Source: CAD feature listing. Evaluate the final solid. Frame: model axes, mm. Face numbers are marked on the shaded views. A direction names the side the tool comes from. Round coordinates to 2 decimals unless told otherwise and drop trailing zeros. Loops run counter-clockwise (first coordinate to the right, second up) from the corner with the lowest first, then second, coordinate; pieces in that order, holes last. Notation, with made-up numbers: M 89,-10.5 L 115,-10.5 A16 cw 115,8.5 Z; hole C 32.5,81 d6. An arc over 180 degrees is marked long. Answer as a JSON object with one key per item and string values.
from build123d import *

# Parameters (mm, degrees)
SKETCH1_W                       = 36
SKETCH1_H                       = 36
BOSS_EXTRUDE1_DEPTH             = 13.5
SKETCH1_3_W                     = 40
SKETCH1_3_H                     = 48.5
SKETCH1_3_W_2                   = 36
SKETCH1_3_H_2                   = 36
BOSS_EXTRUDE2_DEPTH             = 10
FILLET1_R                       = 3.5
FILLET2_R                       = 3.5
FILLET3_R                       = 1
FILLET4_R                       = 1
FILLET5_R                       = 1
BOSS_EXTRUDE3_REACH             = 39.343
BOSS_EXTRUDE3_DIRECTION_2_REACH = 39.343
BOSS_EXTRUDE4_REACH             = 41.68
BOSS_EXTRUDE4_DIRECTION_2_REACH = 41.68
BOSS_EXTRUDE5_DEPTH             = 12.5
SKETCH9_R                       = 2
CUT_EXTRUDE3_DEPTH              = 71.944630699
FILLET6_R                       = 1
FILLET7_R                       = 1


with BuildPart() as part:
    # Sketch1 → Boss-Extrude1 (new body)
    with BuildSketch(Plane.XY):
        Rectangle(SKETCH1_W, SKETCH1_H)
    extrude(amount=BOSS_EXTRUDE1_DEPTH)

    # Fillet2
    fillet2_edges = [part.edges().sort_by_distance(p)[0] for p in [
        (-18, 18, 6.75),
        (-18, -18, 6.75),
        (18, -18, 6.75),
        (18, 18, 6.75),
    ]]
    fillet(fillet2_edges, radius=FILLET2_R)

    # Fillet5
    fillet5_edges = [part.edges().sort_by_distance(p)[0] for p in [
        (0, 18, 13.5),
        (18, 0, 13.5),
        (-18, 0, 13.5),
        (0, -18, 13.5),
        (-16.974873734, 16.974873734, 13.5),
        (-16.974873734, -16.974873734, 13.5),
        (16.974873734, -16.974873734, 13.5),
        (16.974873734, 16.974873734, 13.5),
    ]]
    fillet(fillet5_edges, radius=FILLET5_R)


with BuildPart() as body_2:
    # Sketch1_3 → Boss-Extrude2 (new body)
    # profile 1 of 2: a face of its own
    with BuildSketch(Plane.XY):
        with Locations((0, -4.25)):
            Rectangle(SKETCH1_3_W, SKETCH1_3_H)
        Rectangle(SKETCH1_3_W_2, SKETCH1_3_H_2, mode=Mode.SUBTRACT)
    # profile 2 of 2: a face of its own
    with BuildSketch(Plane.XY):
        Rectangle(SKETCH1_3_W_2, SKETCH1_3_H_2)
    extrude(amount=-BOSS_EXTRUDE2_DEPTH)

    # Fillet1
    fillet1_edges = [body_2.edges().sort_by_distance(p)[0] for p in [
        (20, -28.5, -5),
        (-20, -28.5, -5),
        (-20, 20, -5),
        (20, 20, -5),
    ]]
    fillet(fillet1_edges, radius=FILLET1_R)

    # Fillet3
    fillet3_edges = [body_2.edges().sort_by_distance(p)[0] for p in [
        (20, -4.25, 0),
        (0, 20, 0),
        (-20, -4.25, 0),
        (0, -28.5, 0),
        (-18.974873734, 18.974873734, 0),
        (18.974873734, -27.474873734, 0),
        (-18.974873734, -27.474873734, 0),
        (18.974873734, 18.974873734, 0),
    ]]
    fillet(fillet3_edges, radius=FILLET3_R)

    # Fillet4
    fillet4_edges = [body_2.edges().sort_by_distance(p)[0] for p in [
        (20, -4.25, -10),
        (0, 20, -10),
        (0, -28.5, -10),
        (-20, -4.25, -10),
        (-18.974873734, 18.974873734, -10),
        (18.974873734, -27.474873734, -10),
        (-18.974873734, -27.474873734, -10),
        (18.974873734, 18.974873734, -10),
    ]]
    fillet(fillet4_edges, radius=FILLET4_R)


with BuildPart() as body_3:

    # Boss-Extrude3: up to this face of the body (flat: up to its plane)
    boss_extrude3_end = Plane(body_2.part.faces().sort_by_distance((20, -4.25, -5))[0])
    # Sketch2 → Boss-Extrude3 (new, up to the picked face)
    with BuildSketch(Plane(origin=(0, 0, 0), x_dir=(0, 0, -1), z_dir=(1, 0, 0)), mode=Mode.PRIVATE) as boss_extrude3_sk1:
        Polygon((-2.875, -18), (-2.875, -31.5), (13, -31.5), (13, 20), (13, 23), (-2.875, 23), (-2.875, 18.25), (0.125, 18.25), (0.125, 20), (10, 20), (10, -28.5), (0.125, -28.5), (0.125, -18), align=None)
    boss_extrude3_tool1 = split(extrude(boss_extrude3_sk1.sketch, amount=BOSS_EXTRUDE3_REACH, mode=Mode.PRIVATE), bisect_by=boss_extrude3_end, keep=Keep.BOTH, mode=Mode.PRIVATE)
    add(boss_extrude3_tool1.solids().sort_by(Axis((0, -24.75, 2.30735), (1, 0, 0)))[0])


    # Boss-Extrude3 direction 2: up to this face of the body (flat: up to its plane)
    boss_extrude3_direction_2_end = Plane(body_2.part.faces().sort_by_distance((-20, -4.25, -5))[0])
    # Sketch2 → Boss-Extrude3 direction 2 (add, up to the picked face)
    with BuildSketch(Plane(origin=(0, 0, 0), x_dir=(0, 0, -1), z_dir=(1, 0, 0)), mode=Mode.PRIVATE) as boss_extrude3_direction_2_sk1:
        Polygon((-2.875, -18), (-2.875, -31.5), (13, -31.5), (13, 20), (13, 23), (-2.875, 23), (-2.875, 18.25), (0.125, 18.25), (0.125, 20), (10, 20), (10, -28.5), (0.125, -28.5), (0.125, -18), align=None)
    boss_extrude3_direction_2_tool1 = split(extrude(boss_extrude3_direction_2_sk1.sketch, amount=-BOSS_EXTRUDE3_DIRECTION_2_REACH, mode=Mode.PRIVATE), bisect_by=boss_extrude3_direction_2_end, keep=Keep.BOTH, mode=Mode.PRIVATE)
    add(boss_extrude3_direction_2_tool1.solids().sort_by(Axis((0, -24.75, 2.30735), (-1, 0, 0)))[0])


    # Boss-Extrude4: up to this face of the body (flat: up to its plane)
    boss_extrude4_end = Plane(body_2.part.faces().sort_by_distance((20, -4.25, -5))[0])
    # Sketch3 → Boss-Extrude4 (add, up to the picked face)
    with BuildSketch(Plane(origin=(0, 0, 0), x_dir=(0, 0, -1), z_dir=(1, 0, 0)), mode=Mode.PRIVATE) as boss_extrude4_sk1:
        Polygon((58, -15.625), (10, -15.625), (10, 23), (13, 23), (50, -12.625), (58, -12.625), align=None)
        Polygon((13, 18.835445964), (13, -12.625), (45.674708791, -12.625), align=None, mode=Mode.SUBTRACT)
    boss_extrude4_tool1 = split(extrude(boss_extrude4_sk1.sketch, amount=BOSS_EXTRUDE4_REACH, mode=Mode.PRIVATE), bisect_by=boss_extrude4_end, keep=Keep.BOTH, mode=Mode.PRIVATE)
    add(boss_extrude4_tool1.solids().sort_by(Axis((0, -15.008892, -34), (1, 0, 0)))[0])


    # Boss-Extrude4 direction 2: up to this face of the body (flat: up to its plane)
    boss_extrude4_direction_2_end = Plane(body_2.part.faces().sort_by_distance((-20, -4.25, -5))[0])
    # Sketch3 → Boss-Extrude4 direction 2 (add, up to the picked face)
    with BuildSketch(Plane(origin=(0, 0, 0), x_dir=(0, 0, -1), z_dir=(1, 0, 0)), mode=Mode.PRIVATE) as boss_extrude4_direction_2_sk1:
        Polygon((58, -15.625), (10, -15.625), (10, 23), (13, 23), (50, -12.625), (58, -12.625), align=None)
        Polygon((13, 18.835445964), (13, -12.625), (45.674708791, -12.625), align=None, mode=Mode.SUBTRACT)
    boss_extrude4_direction_2_tool1 = split(extrude(boss_extrude4_direction_2_sk1.sketch, amount=-BOSS_EXTRUDE4_DIRECTION_2_REACH, mode=Mode.PRIVATE), bisect_by=boss_extrude4_direction_2_end, keep=Keep.BOTH, mode=Mode.PRIVATE)
    add(boss_extrude4_direction_2_tool1.solids().sort_by(Axis((0, -15.008892, -34), (-1, 0, 0)))[0])

    # Sketch8 → Boss-Extrude5 (add, symmetric)
    with BuildSketch(Plane(origin=(0, 0, 0), x_dir=(0, 0, -1), z_dir=(1, 0, 0))):
        Polygon((-2.875, -31.5), (-2.875, -33.5), (27.125, -33.5), (27.125, -31.5), (13, -31.5), align=None)
    extrude(amount=BOSS_EXTRUDE5_DEPTH, both=True)

    # Sketch9 → Cut-Extrude3 (cut, through all)
    with BuildSketch(Plane(origin=(0, -12.625, 0), x_dir=(1, 0, 0), z_dir=(0, 1, 0))):
        with Locations(Location((12.7, 54, 0), (0, 0, 270))):
            Circle(SKETCH9_R)
        with Locations(Location((-12.7, 54, 0), (0, 0, 270))):
            Circle(SKETCH9_R)
    extrude(amount=-CUT_EXTRUDE3_DEPTH, mode=Mode.SUBTRACT)

    # Fillet6
    fillet6_edges = [body_3.edges().sort_by_distance(p)[0] for p in [
        (0, 18.25, 2.875),
        (0, 23, 2.875),
        (0, 23, -13),
        (0, -18, 2.875),
        (0, 18.835445964, -13),
        (0, -12.625, -13),
        (0, -12.625, -45.674708791),
    ]]
    fillet(fillet6_edges, radius=FILLET6_R)

    # Fillet7
    fillet7_edges = [body_3.edges().sort_by_distance(p)[0] for p in [
        (-12.5, -33.5, -12.125),
        (0, -33.5, 2.875),
        (0, -33.5, -27.125),
        (12.5, -33.5, -12.125),
    ]]
    fillet(fillet7_edges, radius=FILLET7_R)


solid = body_3.part
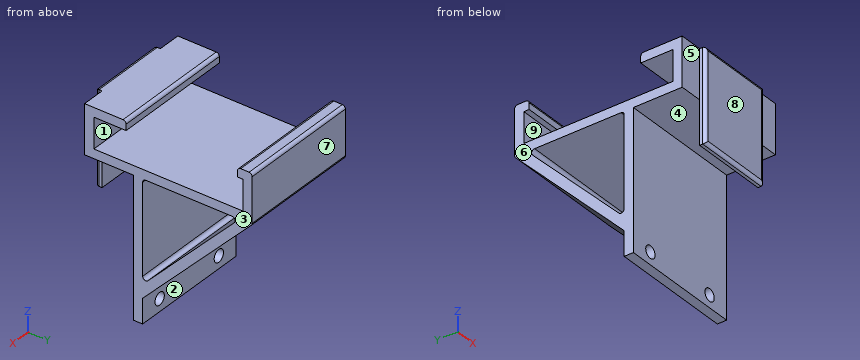
Item 1: Contact query for flat-ended pins moving along their axis: pin 1 Ø1 at (x, y) = (-12, -0.5) entering from -Z; pin 2 Ø12.5 at (x, y) = (-2.5, -22) entering from -Z; pin 3 Ø1.1 at (y, z) = (-32, -13) entering from -X; pin 4 Ø14 at (x, y) = (-3.5, 1) entering from -Z. Output: stop coordinate, or through.
Answer sheet:
{"pin 1": "stops at z = -37.93", "pin 2": "stops at z = -13", "pin 3": "stops at x = -20", "pin 4": "stops at z = -43.12"}
Item 2: Section C-C on y = -13.5. Return the cut outline in (x, z).
Answer sheet:
{"outline": "M -20,-58 L 20,-58 L 20,-10 L -20,-10 Z; hole C -12.7,-54 d4; hole C 12.7,-54 d4"}
Item 3: Access query for the marked faces 1, 2, 3, 4 and 5. Directions: +Z, -Z, +X, -X, +Y, -Y. A direction counts if a zero-diameter tool reaches every point of the face in a straight line with its end or side. Return the directions, or none.
Answer sheet:
{"face 1": "+X, -X", "face 2": "-Z, +X, -X, +Y", "face 3": "+Z, -Z, +X, +Y, -Y", "face 4": "-Z, +X, -X", "face 5": "+Z, -Z, -X, -Y"}
Item 4: Section D-D on z = -32. Return the cut outline in (x, y) (3 decimals).
Answer sheet:
{"outline": "M -20,-15.625 L 20,-15.625 L 20,-12.625 L -20,-12.625 Z; M -20,0.542 L 20,0.542 L 20,4.706 L -20,4.706 Z"}
Item 5: Line query: probe 1 along X at (y, z) = (-13, -54); probe 2 along Y at (x, z) = (-13, -3); probe 3 along Y at (x, z) = (9.5, -18.5) (3 decimals). Output: solid intervals per line, ascending. Write a range as from..to.
Answer sheet:
{"probe 1": "x = -20..-14.7, -10.7..10.7, 14.7..20", "probe 2": "y = -31.5..-28.5, 20..23", "probe 3": "y = -33.5..-31.5, -15.625..-12.625, 13.54..17.704"}
Item 6: Pull-direction query (Y, two-part tool) for the marked faces 6, 7, 8 and 9; classes: pulls with the +Y half, pulls with the -Y half, needs draft (parallel to the pull), parting line crosses it, or undercut.
Answer sheet:
{"face 6": "needs draft", "face 7": "pulls with the +Y half", "face 8": "pulls with the -Y half", "face 9": "undercut"}
Item 7: Section B-B on x = 16.5. Return the cut outline in (y, z) (3 decimals), then the cut area to 3 significant figures.
Answer sheet:
{"outline": "M -31.5,-13 L -15.625,-13 L -15.625,-58 L -12.625,-58 L -12.625,-50 L 22.72,-13.29 A1 ccw 23,-12.597 L 23,1.875 A1 ccw 22,2.875 L 19.25,2.875 A1 ccw 18.25,1.875 L 18.25,-0.125 L 20,-0.125 L 20,-10 L -28.5,-10 L -28.5,-0.125 L -18,-0.125 L -18,1.875 A1 ccw -19,2.875 L -31.5,2.875 Z; hole M -12.625,-43.194 A1 ccw -10.905,-43.888 L 17.205,-14.694 A1 ccw 16.484,-13 L -11.625,-13 A1 ccw -12.625,-14 Z", "area": "560 mm²"}
Item 8: Section A-A on z = -54. Return the cut outline in (x, y) (3 decimals).
Answer sheet:
{"outline": "M -20,-15.625 L -14.7,-15.625 L -14.7,-12.625 L -20,-12.625 Z; M -10.7,-15.625 L 10.7,-15.625 L 10.7,-12.625 L -10.7,-12.625 Z; M 14.7,-15.625 L 20,-15.625 L 20,-12.625 L 14.7,-12.625 Z"}
